from build123d import *

# Parameters (mm, degrees)
F0_W     = 82.55
F0_H     = 25.4
F0_R     = 3.556
F1_DEPTH = 6.35
F2_W     = 25.4
F2_H     = 25.4
F3_DEPTH = 114.3
F5_DEPTH = 25.4
F6_W     = 38.1
F6_H     = 38.1
F6_W_2   = 25.4
F7_DEPTH = 3.81
F9_DEPTH = 25.4
F10_SIZE = 5.08


with BuildPart() as f1:
    # F0 (on Top) → F1 (new body)
    with BuildSketch(Plane.XY):
        Rectangle(F0_W, F0_H)
        with Locations((-34.29, 0)):
            Circle(F0_R, mode=Mode.SUBTRACT)
        with Locations((34.29, 0)):
            Circle(F0_R, mode=Mode.SUBTRACT)
    extrude(amount=F1_DEPTH)

    # F2 (on face) → F3 (join)
    with BuildSketch(Plane.XY.offset(6.35)):
        Rectangle(F2_W, F2_H)
    extrude(amount=F3_DEPTH)

    # F4 (on face) → F5 (cut)
    with BuildSketch(Plane.YZ.offset(12.7)):
        Polygon((12.7, 120.65), (-12.7, 120.65), (12.7, 81.5374299191), align=None)
    extrude(amount=-F5_DEPTH, mode=Mode.SUBTRACT)

    # F6 (on face) → F7 (join)
    with BuildSketch(Plane(origin=(0, 46.1768520488, 29.9875983504), x_dir=(-1, 0, 0), z_dir=(0, 0.8386705679, 0.544639035))):
        with Locations((-31.75, 80.5161269144)):
            Rectangle(F6_W, F6_H)
        with Locations((0, 80.5161269144)):
            Rectangle(F6_W_2, F6_H)
        with Locations((31.75, 80.5161269144)):
            Rectangle(F6_W, F6_H)
    extrude(amount=F7_DEPTH)

    # F8 (on face) → F9 (cut)
    with BuildSketch(Plane.YZ.offset(12.7)):
        Polygon((-12.7, 110.4715185089), (-8.0507472341, 113.4907785578), (-12.7, 120.65), align=None)
    extrude(amount=-F9_DEPTH, mode=Mode.SUBTRACT)

    # F10
    f10_edges = [f1.edges().sort_by_distance(p)[0] for p in [
        (12.7, 0, 6.35),
        (-12.7, 0, 6.35),
        (12.7, 2.324626, 97.514104),
        (-12.7, 2.324626, 97.514104),
    ]]
    chamfer(f10_edges, length=F10_SIZE)


solid = f1.part
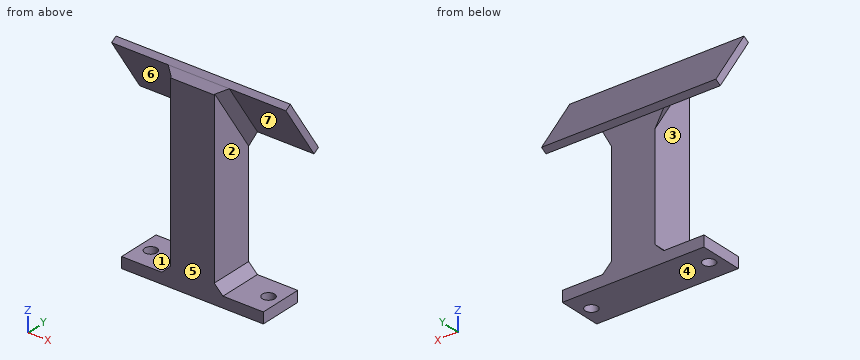
Could you check a few things on this model? Use its own coordinates, in mm. Face numbers are marked on the shaded views. A direction names the side the tool comes from. Round coordinates to 2 decimals unless told otherwise and drop trailing zeros. Order: outer loops, then holes, each group sorted by start corner. A loop starts at its lowest first (then second) coordinate and runs counter-clockwise, first axis right, second up. Notation, with made-up numbers: M -23.75,47 L -16.75,47 A27 ccw -16.75,86 Z; hole C -15,11.5 d2. An arc over 180 degrees is marked long. One line per item, written item: value.
(1) Imagine slicing it at C-C (x = -34.29). Write out the boundary of the cut face in (y, z), and give its area (3 significant figures).
Ans:
outline: M -12.7,0 L -3.56,0 L -3.56,6.35 L -12.7,6.35 Z; M -8.05,113.49 L 12.7,81.54 L 15.9,83.61 L -4.86,115.57 Z; M 3.56,0 L 12.7,0 L 12.7,6.35 L 3.56,6.35 Z
area: 261 mm^2
(2) Imagine slicing it at D-D (z = 91). Write out the boundary of the cut face in (x, y).
Ans:
outline: M -50.8,6.55 L -17.78,6.55 L -12.7,0.5 L -12.7,-12.7 L 12.7,-12.7 L 12.7,0.5 L 17.78,6.55 L 50.8,6.55 L 50.8,11.1 L -50.8,11.1 Z
(3) Imagine slicing it at A-A (x = -21). Write out the boundary of the cut face in (y, z), and give its area (3 significant figures).
Ans:
outline: M -12.7,0 L 12.7,0 L 12.7,6.35 L -12.7,6.35 Z; M -8.05,113.49 L 12.7,81.54 L 15.9,83.61 L -4.86,115.57 Z
area: 306 mm^2
(4) Imagine slicing it at B-B (y = 0). Write out the boundary of the cut face in (x, z) (3 decimals), and give its area (3 significant figures).
Ans:
outline: M -50.8,101.094 L -17.78,101.094 L -12.7,91.766 L -12.7,11.43 L -17.78,6.35 L -30.734,6.35 L -30.734,0 L 30.734,0 L 30.734,6.35 L 17.78,6.35 L 12.7,11.43 L 12.7,91.766 L 17.78,101.094 L 50.8,101.094 L 50.8,108.089 L -50.8,108.089 Z; M -41.275,0 L -37.846,0 L -37.846,6.35 L -41.275,6.35 Z; M 37.846,0 L 41.275,0 L 41.275,6.35 L 37.846,6.35 Z
area: 3,620 mm^2
(5) Which directions (+Z, -Z, +X, -X, +Y, -Y) give clear straight access to the entire face, cutting with the end or side of a thin tool? Please do the marked faces 1, 2 and 3.
Ans:
face 1: -X, +Y, -Y
face 2: +X, -Y
face 3: -X, -Y
(6) I'm going to push flat-ended pins straight in: P1, Ø1.5, axis at y = 4.5, z = 22, coming from the -X side; P2, Ø6.5, axis at x = 34.29, y = 0, coming from the -Z side; P3, Ø2, axis at x = -6.5, z = 15.5, coming from the +Y side. Where does each tip first touch, or does it pass through?
Ans:
P1: stops at x = -12.7
P2: stops at z = 96.09
P3: stops at y = 12.7
(7) I need wall thicknesses on line 1 along Y through (x, z) = (-34, 1); line 2 along Y through (x, z) = (34.29, 4.5); line 3 along Y through (x, z) = (0, 22.5). Which ranges of each line are inside material? Lowest first, please. Write a range as from..to.
Ans:
line 1: y = -12.7..-3.54, 3.54..12.7
line 2: y = -12.7..-3.56, 3.56..12.7
line 3: y = -12.7..12.7
(8) If we mould it in two halves opening along Z, with no side actions, what happens to the marked faces 4, 5, 6 and 7? For each: released by +Z, released by -Z, zero draft, split by the parting line, or undercut.
Ans:
face 4: released by -Z
face 5: zero draft
face 6: undercut
face 7: undercut
